Design review of the part shown in the three views and the two pictorial views. Dimensions are in mm from the part's minimum x, y and z. A direction names the side the tool comes from. Round coordinates to 2 decimals unless told otherwise and drop trailing zeros. Order: outer loops, then holes, each group sorted by start corner. A loop starts at its lowest first (then second) coordinate and runs counter-clockwise, first axis right, second up. Notation, with made-up numbers: (14.25, 27.25) -> (39.25, 27.25) arc R11 cw to (39.25, 45.25) -> close; hole circle Ø9 at (-13, 58.25). An arc over 180 degrees is marked (long way). Put each result on its own line as item: value. Start each with the question number.
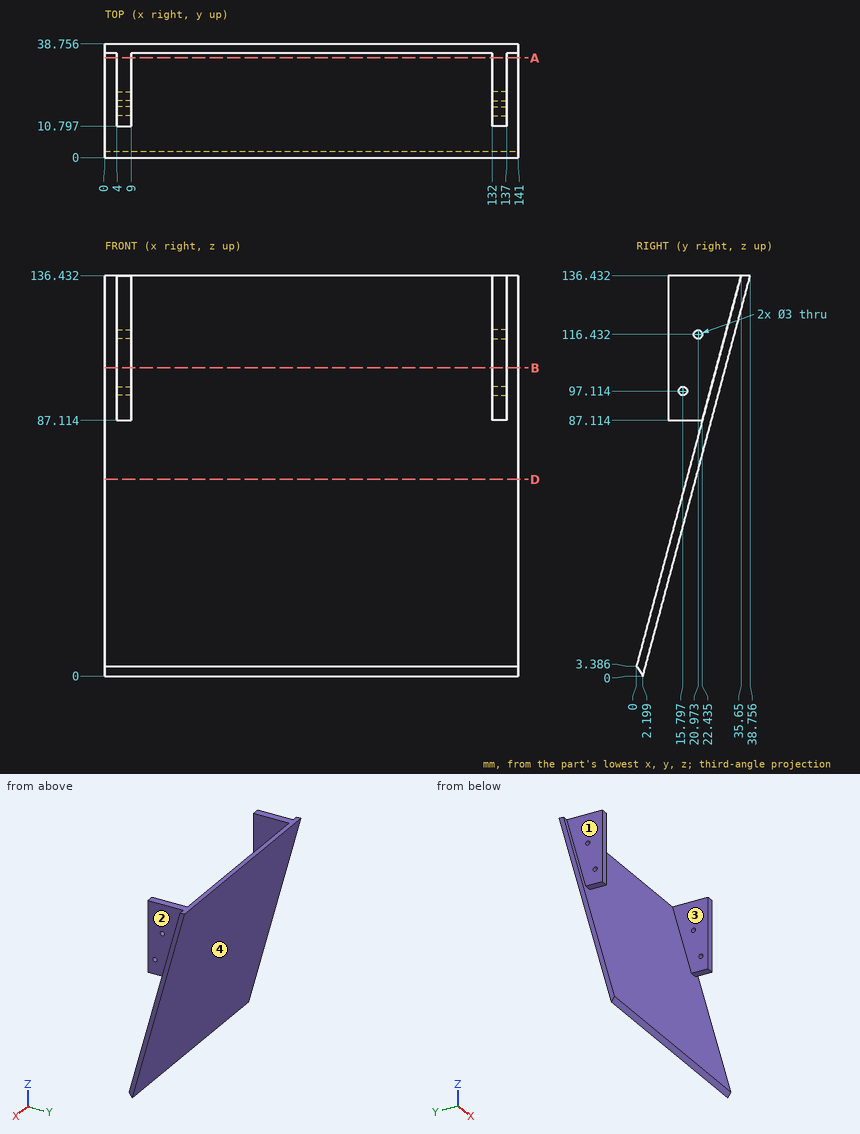
Q1. Take a section at B-B on z = 105. Give the boundary of the cut face in (x, y).
Q2. For the marked faces 1, 2, 3 and 4, list the 3-axis set-ups (+Z, -Z, +X, -X, +Y, -Y) from which the entire face can be reached by the end or side of a thin tool; tool diameter is ignored.
Q3. Clearance check with flat-ended pins moving along their axes: pin 1 Ø1.5 at (x, z) = (109, 19) entering from -Y; pin 2 Ø5 at (x, z) = (19, 67) entering from +Y; pin 3 Ø4 at (x, z) = (134, 115) entering from -Y; pin 4 Ø4 at (y, z) = (9.5, 47) entering from +X. State where each tip first meets the part, or that it passes through.
Q4. Wall thickness on probe 1 along X at (y, z) = (17, 123.5); probe 2 along Y at (x, z) = (89, 62.5) (1 decimal); probe 3 along Y at (x, z) = (36, 126) (1 decimal): over which ranges is each line inside the solid? List them lowest first. Write a range as [from, to].
Q5. Take a section at A-A on y = 34. Give the boundary of the cut face in (x, z) (1 decimal).
Q6. Take a section at D-D on z = 67. Give the boundary of the cut face in (x, y) (1 decimal).
Calculated:
1. outline: (0, 27.23) -> (4, 27.23) -> (4, 10.8) -> (9, 10.8) -> (9, 27.23) -> (132, 27.23) -> (132, 10.8) -> (137, 10.8) -> (137, 27.23) -> (141, 27.23) -> (141, 30.33) -> (0, 30.33) -> close
2. face 1: +Z, -X, -Y
2. face 2: +Z, +X, -Y
2. face 3: +Z, -Y
2. face 4: -Z, +X, -X, +Y
3. pin 1: stops at y = 3.98
3. pin 2: stops at y = 20.82
3. pin 3: stops at y = 10.8
3. pin 4: passes through
4. probe 1: x = [4, 9], [132, 137]
4. probe 2: y = [15.8, 18.9]
4. probe 3: y = [32.9, 36]
5. outline: (0, 118.7) -> (141, 118.7) -> (141, 130.3) -> (137, 130.3) -> (137, 136.4) -> (132, 136.4) -> (132, 130.3) -> (9, 130.3) -> (9, 136.4) -> (4, 136.4) -> (4, 130.3) -> (0, 130.3) -> close
6. outline: (0, 17) -> (141, 17) -> (141, 20.2) -> (0, 20.2) -> close
